from build123d import *

# Parameters (mm, degrees)
SZKIC1_R                    = 15
DODANIE_WYCI_GNI_CIE1_DEPTH = 20
SKETCH1_R                   = 9.385297187
CUT_EXTRUDE1_DEPTH          = 34
CUT_EXTRUDE1_DEPTH_BACK     = 23


with BuildPart() as part:
    # Szkic1 → Dodanie-wyciągnięcie1 (new body, symmetric)
    with BuildSketch(Plane(origin=(0, 0, 0), x_dir=(0, 0, -1), z_dir=(1, 0, 0))):
        Circle(SZKIC1_R)
    extrude(amount=DODANIE_WYCI_GNI_CIE1_DEPTH, both=True)

    # Sketch1 → Cut-Extrude1 (cut, two sides)
    with BuildSketch(Plane(origin=(0, 0, 0), x_dir=(1, 0, 0), z_dir=(0, 1, 0))) as cut_extrude1_sk:
        with Locations(Location((0, 0, 0), (0, 0, 90))):  # turned: the seam where the file's is
            Circle(SKETCH1_R)
    extrude(amount=CUT_EXTRUDE1_DEPTH, mode=Mode.SUBTRACT)
    extrude(cut_extrude1_sk.sketch, amount=-CUT_EXTRUDE1_DEPTH_BACK, mode=Mode.SUBTRACT)

    # Sketch2 → Cut-Revolve1 (revolve, cut)
    with BuildSketch(Plane(origin=(0, 0, 0), x_dir=(0, 0, -1), z_dir=(1, 0, 0)), mode=Mode.PRIVATE) as cut_revolve1_sk:
        Polygon((0, 2.315822277), (0, 32.756739461), (-30.440917184, 32.756739461), align=None)
    revolve(cut_revolve1_sk.sketch.rotate(Axis((0, 2.315822277, 0), (0, 1, 0)), 180), axis=Axis((0, 2.315822277, 0), (0, 1, 0)), mode=Mode.SUBTRACT)  # turned: the seam where the file's is


solid = part.part
Could you check a few things on this model? Use its own coordinates, in mm. A direction names the side the tool comes from. Give positions to 0.01 mm unless a question says otherwise; leave off trailing zeros. Order: outer loops, then holes, each group sorted by start corner. A loop starts at its lowest first (then second) coordinate and runs counter-clockwise, first axis right, second up. Notation, with made-up numbers: (9.5, 35) -> (59.5, 35) arc R26 ccw to (59.5, 53) -> close; hole circle Ø7 at (-18, 77.5). An arc over 180 degrees is marked (long way). Return JSON: item names as keys, results as strings.
1. On a 3-axis mill with a long thin cutter (end or side, diameter ignored), from which of +Z, -Z, +X, -X, +Y, -Y can I reach the whole of each face in a straight line? I mean faces 5 (the conical face through (9.91, 12.23, 0.22)), 6 (the flat face through (20, 0, 0)). Say none if no direction works.
Answer list:
{"face 5": "+Y", "face 6": "+Z, -Z, +X, +Y, -Y"}
2. Imagine slicing it at D-D on y = 0. List the corners of the cut face in (x, z) for me, then the cut area to 3 significant figures.
Answer list:
{"outline": "(-20, -15) -> (20, -15) -> (20, 15) -> (-20, 15) -> close; hole circle Ø18.77 at (0, 0)", "area": "923 mm2"}
3. Thinking about a two-plate mould opening in Z: for faces 1 (the flat face through (-20, 0, 0)), 2 (the conical face through (-9.91, 12.23, -0.22)), 3 (the cylindrical face through (-2.82, -1.47, -8.95)), 4 (the cylindrical face through (0, -9, 12)), which applies, pulls with the +Z half, pulls with the -Z half, needs draft (parallel to the pull), parting line crosses it, or undercut?
Answer list:
{"face 1": "needs draft", "face 2": "undercut", "face 3": "undercut", "face 4": "parting line crosses it"}
4. Imagine slicing it at A-A on y = 9. List the corners of the cut face in (x, z) for me.
Answer list:
{"outline": "(-20, -12) -> (20, -12) -> (20, 12) -> (-20, 12) -> close; hole circle Ø18.77 at (0, 0)"}
5. Imagine slicing it at B-B on z = 0. List the corners of the cut face in (x, y) for me, then the cut area to 3 significant figures.
Answer list:
{"outline": "(-20, -15) -> (-9.39, -15) -> (-9.39, 11.7) -> (-12.68, 15) -> (-20, 15) -> close; (9.39, -15) -> (20, -15) -> (20, 15) -> (12.68, 15) -> (9.39, 11.7) -> close", "area": "626 mm2"}
6. Imagine slicing it at C-C on x = 15.5. List the corners of the cut face in (y, z) for me.
Answer list:
{"outline": "circle Ø30 at (0, 0)"}
7. For pin 1 Ø1.5 at (x, y) = (10, -6.5) entering from -Z; pin 2 Ø1 at (x, y) = (5.5, 8.5) entering from -Z; pin 3 Ø3 at (x, z) = (-10, 11) entering from +Y, each with a flat end and sliding along its axis, tell me the tip position at first contact or that it passes through.
Answer list:
{"pin 1": "stops at z = -13.85", "pin 2": "stops at z = -12.69", "pin 3": "stops at y = 11.61"}
8. I need wall thicknesses on line 1 (X direction, y = 0, z = 0); line 2 (Z direction, x = -6.5, y = -4); line 3 (X direction, y = -5, z = -2.5). Which ranges of each line are inside material? Lowest first, please. Write a range as from..to.
Answer list:
{"line 1": "x = -20..-9.39, 9.39..20", "line 2": "z = -14.46..-6.77, 6.77..14.46", "line 3": "x = -20..-9.05, 9.05..20"}
